Check sheet for the modelled part. Datum: model origin and axes. Units: mm. A direction names the side the tool comes from. Round coordinates to 2 decimals unless told otherwise and drop trailing zeros. Order: outer loops, then holes, each group sorted by start corner. A loop starts at its lowest first (then second) coordinate and runs counter-clockwise, first axis right, second up.
```python
from build123d import *

# Parameters (mm, degrees)
SKICA1_R                = 3
P_IDAT_VYSUNUT_M2_DEPTH = 7


with BuildPart() as part:
    # Skica1 → Přidat vysunutím2 (new body)
    with BuildSketch(Plane.XY):
        with BuildLine():
            Line((40.64, 24.256759883), (-2.88, 7.463618425))
            ThreePointArc((-2.88, 7.463618425), (-8, 0), (-2.88, -7.463618425))
            Line((-2.88, -7.463618425), (34.015875108, -21.700696777))
            ThreePointArc((34.015875108, -21.700696777), (35.406329056, -21.719066966), (36.472668864, -20.82653178))
            ThreePointArc((36.472668864, -20.82653178), (40.594655389, -10.773762289), (42, 0))
            ThreePointArc((42, 0), (50, 8), (58, 0))
            ThreePointArc((58, 0), (56.838027177, -11.55156555), (53.398666667, -22.640282644))
            ThreePointArc((53.398666667, -22.640282644), (53.703822927, -24.701669361), (55.676666667, -25.37273055))
            ThreePointArc((55.676666667, -25.37273055), (74.88299251, 7.539010793), (40.64, 24.256759883))
        make_face()
        Circle(SKICA1_R, mode=Mode.SUBTRACT)
    extrude(amount=P_IDAT_VYSUNUT_M2_DEPTH)


solid = part.part
```
Item 1: Release check for a two-part mould opening along Y. For faces 1 (the cylindrical face through (50, 8, 3)), 2 (the flat face through (33, 1, 7)), 3 (the cylindrical face through (75.05, 6.96, 3.45)), 4 (the cylindrical face through (-3, 0, 3)) record: released by +Y, released by -Y, zero draft, split by the parting line, or undercut.
Answer:
face 1: undercut
face 2: zero draft
face 3: split by the parting line
face 4: undercut
Item 2: Access from +Z, -Z, +X, -X, +Y, -Y to the whole of each face (thin tool, end or side, straight path). Record for faces 5 (the flat face through (15.31, -14.482, 3.451)), 6 (the cylindrical face through (56.87, -11.39, 3.45)), 7 (the cylindrical face through (40.555, -10.921, 3.451)).
Answer:
face 5: +Z, -Z, -X, -Y
face 6: +Z, -Z
face 7: +Z, -Z, -Y
Item 3: Sectioned sample at C-C (y = -9). Record the cut outline in (x, z).
Answer:
outline: (1.1, 0) - (41.02, 0) - (41.02, 7) - (1.1, 7) - close; (57.3, 0) - (74.39, 0) - (74.39, 7) - (57.3, 7) - close
Item 4: Go/stop test with flat-tipped pins: P1, Ø2, axis at x = 66, z = 2, coming from the +Y side; P2, Ø2, axis at x = 25, y = -19.5, coming from the +Z side; P3, Ø1, axis at x = 50.5, z = 4, coming from the +Y side. Record where each tip stops, or that it passes through.
Answer:
P1: stops at y = 21.24
P2: passes through
P3: stops at y = 26
Item 5: Scan lines: line 1 along X through (y, z) = (-1, 5.5); line 2 along X through (y, z) = (7, 4); line 3 along Y through (x, z) = (0, 3.25). Record each from-to range of solid material in increasing order.
Answer:
line 1: x = -7.94 to -2.83, 2.83 to 41.99, 57.99 to 75.98
line 2: x = -3.87 to 46.13, 53.87 to 75.04
line 3: y = -8.57 to -3, 3 to 8.57
Item 6: Sectioned sample at B-B (z = 3.75). Record the cut outline in (x, y).
Answer:
outline: (-2.88, -7.46) - (34.02, -21.7) arc R2 ccw to (36.47, -20.83) arc R42 ccw to (42, 0) arc R8 cw to (58, 0) arc R58 cw to (53.4, -22.64) arc R2 ccw to (55.68, -25.37) arc R26 ccw (long way) to (40.64, 24.26) - (-2.88, 7.46) arc R8 ccw to start; hole circle Ø6 at (0, 0)
Item 7: Sectioned sample at D-D (x = 50). Record the cut outline in (y, z), and give its area (3 significant figures).
Answer:
outline: (8, 0) - (26, 0) - (26, 7) - (8, 7) - close
area: 126 mm2
Item 8: Sectioned sample at A-A (x = 1). Record the cut outline in (y, z).
Answer:
outline: (-8.96, 0) - (-2.83, 0) - (-2.83, 7) - (-8.96, 7) - close; (2.83, 0) - (8.96, 0) - (8.96, 7) - (2.83, 7) - close
